from build123d import *

# Parameters (mm, degrees)
F0_W     = 200
F0_H     = 100
F1_DEPTH = 7.4
F2_W     = 8
F2_H     = 2.7
F3_DEPTH = 2
F4_W     = 108
F4_H     = 50
F5_DEPTH = 7.401


with BuildPart() as f1:
    # F0 (on Front) → F1 (new body)
    with BuildSketch(Plane.XZ):
        with Locations((2.203826, 6.35675)):
            Rectangle(F0_W, F0_H)
    extrude(amount=F1_DEPTH)

    # F2 (on face) → F3 (join)
    with BuildSketch(Plane.XZ.offset(7.4)):
        with Locations((-93.796174, 55.00675)):
            Rectangle(F2_W, F2_H)
        with Locations((98.203826, 55.00675)):
            Rectangle(F2_W, F2_H)
        with Locations((98.203826, -42.29325)):
            Rectangle(F2_W, F2_H)
        with Locations((-93.796174, -42.29325)):
            Rectangle(F2_W, F2_H)
    extrude(amount=F3_DEPTH)

    # F4 (on face) → F5 (cut, through all)
    with BuildSketch(Plane.XZ.offset(7.4)):
        Rectangle(F4_W, F4_H)
    extrude(amount=-F5_DEPTH, mode=Mode.SUBTRACT)


solid = f1.part
Work out the finished part from the listing and answer in its coordinate system (mm). A direction names the side the tool comes from. Round coordinates to 2 decimals unless told otherwise and drop trailing zeros. Order: outer loops, then holes, each group sorted by start corner. A loop starts at its lowest first (then second) coordinate and runs counter-clockwise, first axis right, second up. Notation, with made-up numbers: M 12.25,-20.75 L 41.25,-20.75 A34 cw 41.25,11.25 Z; hole C 47,26.25 d1. An arc over 180 degrees is marked long. Put each result on its own line as item: value. Start each with the question number.
Q1. A flat-ended cylindrical pin translates along its axis: pin 1 (3 mm diameter, centred on x = 12.5, z = 41.5, fed in from -Y). Find the tip coordinate at first contact, or state that the pin passes through.
Q2. Section C-C, the plane y = -2.5 is taken. Write down the section's boundary in (x, z), and give its area (3 significant figures).
Q3. A tool of negligible diameter and unlimited length cuts with its end or side. For faces 1 (the flat face through (1, -4, 56.357)), 2 (the flat face through (-1, -4, -25)), from which of +Z, -Z, +X, -X, +Y, -Y can it reach the whole face along a straight path? Write none if from no direction.
Q4. For a pull along Z with two mould halves and no side action, classify faces 3 (the flat face through (1, -4, -43.643)), 4 (the flat face through (-1, -4, 25)), 5 (the flat face through (1, 0, 29)) as pulls with the +Z half, pulls with the -Z half, needs draft (parallel to the pull), parting line crosses it, or undercut.
Q5. Straight lines are drawn through the part: L1, parallel to X at y = -5.25, z = -17; L2, parallel to Z at x = -23.5, y = -2; L3, parallel to Y at x = 68, z = 12. For each, find the intervals that lie inside material, in ascending order. Write a range as [from, to].
Q6. Section B-B, the plane x = -34.5 is taken. Write down the section's boundary in (y, z), and give its area (3 significant figures).
Q7. Section D-D, the plane x = -57 is taken. Write down the section's boundary in (y, z), and give its area (3 significant figures).
Q8. Section A-A, the plane z = -13.5 is taken. Write down the section's boundary in (x, y).
Findings below:
1. pin 1: stops at y = -7.4
2. outline: M -97.8,-43.64 L 102.2,-43.64 L 102.2,56.36 L -97.8,56.36 Z; hole M -54,-25 L 54,-25 L 54,25 L -54,25 Z
2. area: 14,600 mm^2
3. face 1: +Z, +X, -X, +Y, -Y
3. face 2: +Y, -Y
4. face 3: pulls with the -Z half
4. face 4: undercut
4. face 5: needs draft
5. L1: x = [-97.8, -54], [54, 102.2]
5. L2: z = [-43.64, -25], [25, 56.36]
5. L3: y = [-7.4, 0]
6. outline: M -7.4,-43.64 L 0,-43.64 L 0,-25 L -7.4,-25 Z; M -7.4,25 L 0,25 L 0,56.36 L -7.4,56.36 Z
6. area: 370 mm^2
7. outline: M -7.4,-43.64 L 0,-43.64 L 0,56.36 L -7.4,56.36 Z
7. area: 740 mm^2
8. outline: M -97.8,-7.4 L -54,-7.4 L -54,0 L -97.8,0 Z; M 54,-7.4 L 102.2,-7.4 L 102.2,0 L 54,0 Z
